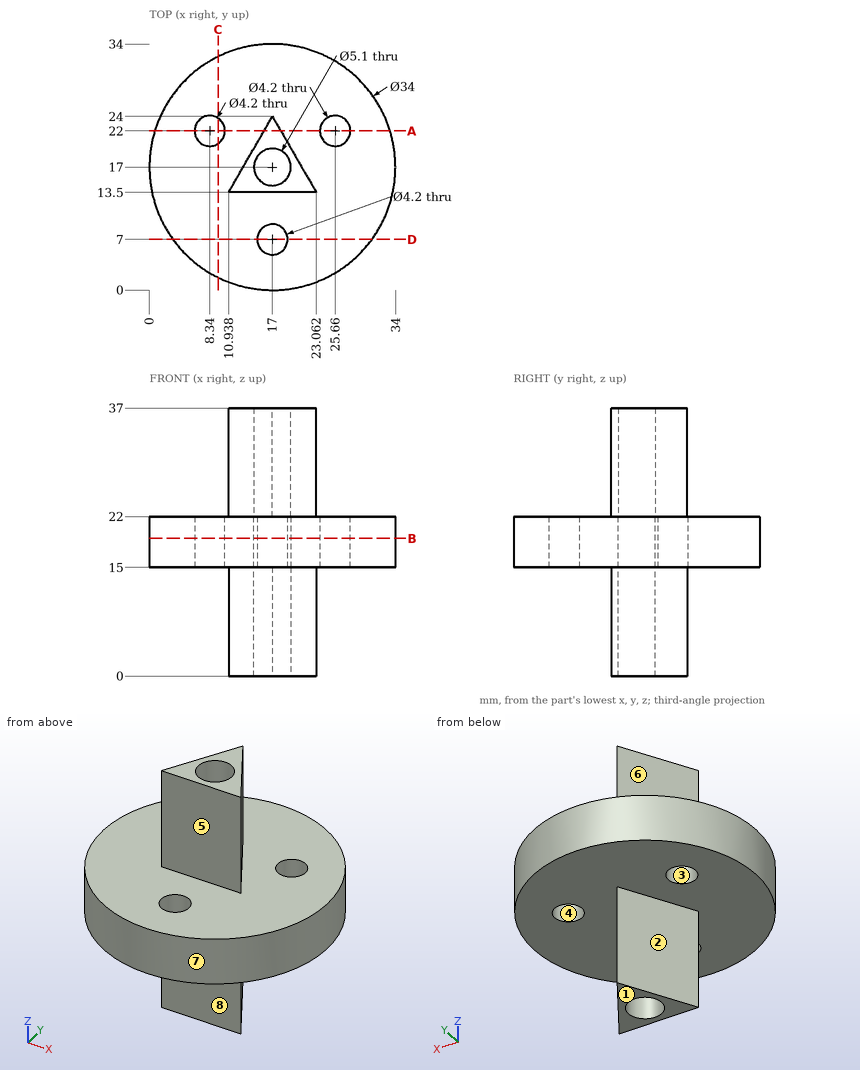
Geometry check sheet. Reference: drawing and pictorial views, mm from the part's lowest x, y, z. A direction names the side the tool comes from. Coordinates: 2 decimals unless noted, no trailing zeros. Order: outer loops, then holes, each group sorted by start corner. A loop starts at its lowest first (then second) coordinate and runs counter-clockwise, first axis right, second up. Notation, with made-up numbers: (65, 4.25) -> (77, 4.25) arc R30 cw to (77, 26.25) -> close; hole circle Ø1 at (-13.5, 6.5). An arc over 180 degrees is marked (long way). Write item = value, one per line. Start each with the question number.
1) Mould release check, pull along Y, two halves, no side actions. Record for the marked faces 1, 2, 3 and 4: +Y half, -Y half, draft (parallel to the pull), parting line (faces both ways), or undercut.
2) Cross-section at C-C (x = 9.5). Enter the section's corners in (y, z).
3) Cross-section at A-A (y = 22). Enter the section's corners in (x, z) (1 decimal).
4) Cross-section at D-D (y = 7). Enter the section's corners in (x, z), then the cut area to 3 significant figures.
5) Material ranges on L1, parallel to Y at x = 17, z = 16; L2, parallel to X at y = 20.5, z = 18.5 (1 decimal); L3, parallel to Z at x = 8, y = 30, recorded low to high.
6) Access from +Z, -Z, +X, -X, +Y, -Y to the whole of each face (thin tool, end or side, straight path). Record for the marked faces 5, 6, 7 and 8.
7) Go/stop test with flat-tipped pins: P1, Ø6, axis at x = 16.5, z = 9.5, coming from the -Y side; P2, Ø8, axis at y = 15.5, z = 30, coming from the +X side; P3, Ø3, axis at x = 17.5, y = 24.5, coming from the -Z side; P4, Ø3, axis at y = 18.5, z = 3.5, coming from the -X side. Record where each tip stops, or that it passes through.
8) Cross-section at B-B (z = 19). Enter the section's corners in (x, y).
Ans:
q1.face_1 = draft
q1.face_2 = +Y half
q1.face_3 = undercut
q1.face_4 = undercut
q2.outline = (1.74, 15) -> (20.25, 15) -> (20.25, 22) -> (1.74, 22) -> close; (23.75, 15) -> (32.26, 15) -> (32.26, 22) -> (23.75, 22) -> close
q3.outline = (0.8, 15) -> (6.2, 15) -> (6.2, 22) -> (0.8, 22) -> close; (10.4, 15) -> (15.8, 15) -> (15.8, 0) -> (18.2, 0) -> (18.2, 15) -> (23.6, 15) -> (23.6, 22) -> (18.2, 22) -> (18.2, 37) -> (15.8, 37) -> (15.8, 22) -> (10.4, 22) -> close; (27.8, 15) -> (33.2, 15) -> (33.2, 22) -> (27.8, 22) -> close
q4.outline = (3.25, 15) -> (14.9, 15) -> (14.9, 22) -> (3.25, 22) -> close; (19.1, 15) -> (30.75, 15) -> (30.75, 22) -> (19.1, 22) -> close
q4.area = 163 mm²
q5.L1 = 0 to 4.9, 9.1 to 14.45, 19.55 to 34
q5.L2 = 0.4 to 6.9, 9.8 to 24.2, 27.1 to 33.6
q5.L3 = 15 to 22
q6.face_5 = +Z, +X, -X, -Y
q6.face_6 = +Z, -X, +Y
q6.face_7 = +Z, -Z
q6.face_8 = -Z, +X, -X, -Y
q7.P1 = 13.5
q7.P2 = 23.06
q7.P3 = 0
q7.P4 = 12.96
q8.outline = circle Ø34 at (17, 17); hole circle Ø4.2 at (8.34, 22); hole circle Ø5.1 at (17, 17); hole circle Ø4.2 at (17, 7); hole circle Ø4.2 at (25.66, 22)
